Geometry: final body of the model. Coordinates: model frame, mm. A direction names the side the tool comes from. Coordinates: 2 decimals unless noted, no trailing zeros. Loops run counter-clockwise (first coordinate to the right, second up) from the corner with the lowest first, then second, coordinate; pieces in that order, holes last. Notation, with made-up numbers: (73, -30) -> (77, -30) arc R29 cw to (77, -2) -> close; hole circle Ø7 at (28.5, -22). An arc over 180 degrees is marked (long way). One line per item, written item: value. Start each with the question number.
Item 1: Contact query for flat-ended pins moving along their axis: pin 1 Ø1.5 at (y, z) = (-2, 3) entering from -X; pin 2 Ø6 at (x, y) = (-2, 11.5) entering from -Z; pin 3 Ø2 at (x, y) = (11.5, 4) entering from +Z; pin 4 Ø1.2 at (x, z) = (1.5, 1.5) entering from -Y. Output: stop coordinate, or through.
Item 2: Section query D-D on y = 5. Return loops of the section in (x, z), then the cut area to 3 significant figures.
Item 3: Section query C-C on z = 2.3. Return loops of the section in (x, y), then the cut area to 3 significant figures.
Item 4: Ray query, probe 1 along Y at (x, z) = (-0.25, 2.45); probe 2 along Z at (x, y) = (2, 12.5); probe 3 along Y at (x, z) = (3.5, 2.1). Return the intervals inside material, ascending. Write a range as from..to.
Item 5: Mould query, pull axis Y, two halves, no side actions, for faces 4 (the flat face through (4.1, 0, 2)), 5 (the flat face through (6.5, -6.5, 1)), 6 (the flat face through (-4.1, 0, 2)), 7 (the cylindrical face through (-14.985, 0.66, 0.493)). Classes: +Y half, -Y half, draft (parallel to the pull), parting line (faces both ways), or undercut.
Item 6: Set-up query: faces 1 (the flat face through (6, 0, 0)), 2 (the cylindrical face through (-7.1, -5.45, 2.48)), 3 (the flat face through (0, 4.1, 2)). Return all of +Z, -Z, +X, -X, +Y, -Y with unobstructed straight access to the full face (end or side cutting, diameter ignored); none if empty.
Item 7: Section query A-A on x = 0. Return loops of the section in (y, z).
from build123d import *

# Parameters (mm, degrees)
SKETCH_R     = 8.95
SKETCH_W     = 8.2
SKETCH_H     = 8.2
PAD_DEPTH    = 4
SKETCH001_R  = 15
SKETCH001_W  = 8.2
SKETCH001_H  = 8.2
PAD001_DEPTH = 1


with BuildPart() as part:
    # Sketch → Pad (new body)
    with BuildSketch(Plane.XY):
        Circle(SKETCH_R)
        Rectangle(SKETCH_W, SKETCH_H, mode=Mode.SUBTRACT)
    extrude(amount=PAD_DEPTH)

    # Sketch001 → Pad001 (join)
    with BuildSketch(Plane.XY):
        Circle(SKETCH001_R)
        Rectangle(SKETCH001_W, SKETCH001_H, mode=Mode.SUBTRACT)
    extrude(amount=PAD001_DEPTH)


solid = part.part
Reply:
1. pin 1: stops at x = -8.86
1. pin 2: stops at z = 0
1. pin 3: stops at z = 1
1. pin 4: stops at y = -14.95
2. outline: (-14.14, 0) -> (14.14, 0) -> (14.14, 1) -> (7.42, 1) -> (7.42, 4) -> (-7.42, 4) -> (-7.42, 1) -> (-14.14, 1) -> close
2. area: 72.8 mm²
3. outline: circle Ø17.9 at (0, 0); hole (-4.1, -4.1) -> (4.1, -4.1) -> (4.1, 4.1) -> (-4.1, 4.1) -> close
3. area: 184 mm²
4. probe 1: y = -8.95..-4.1, 4.1..8.95
4. probe 2: z = 0..1
4. probe 3: y = -8.24..-4.1, 4.1..8.24
5. face 4: undercut
5. face 5: draft
5. face 6: undercut
5. face 7: parting line
6. face 1: -Z, +X, -X, +Y, -Y
6. face 2: +Z
6. face 3: +Z, -Z
7. outline: (-15, 0) -> (-4.1, 0) -> (-4.1, 4) -> (-8.95, 4) -> (-8.95, 1) -> (-15, 1) -> close; (4.1, 0) -> (15, 0) -> (15, 1) -> (8.95, 1) -> (8.95, 4) -> (4.1, 4) -> close
